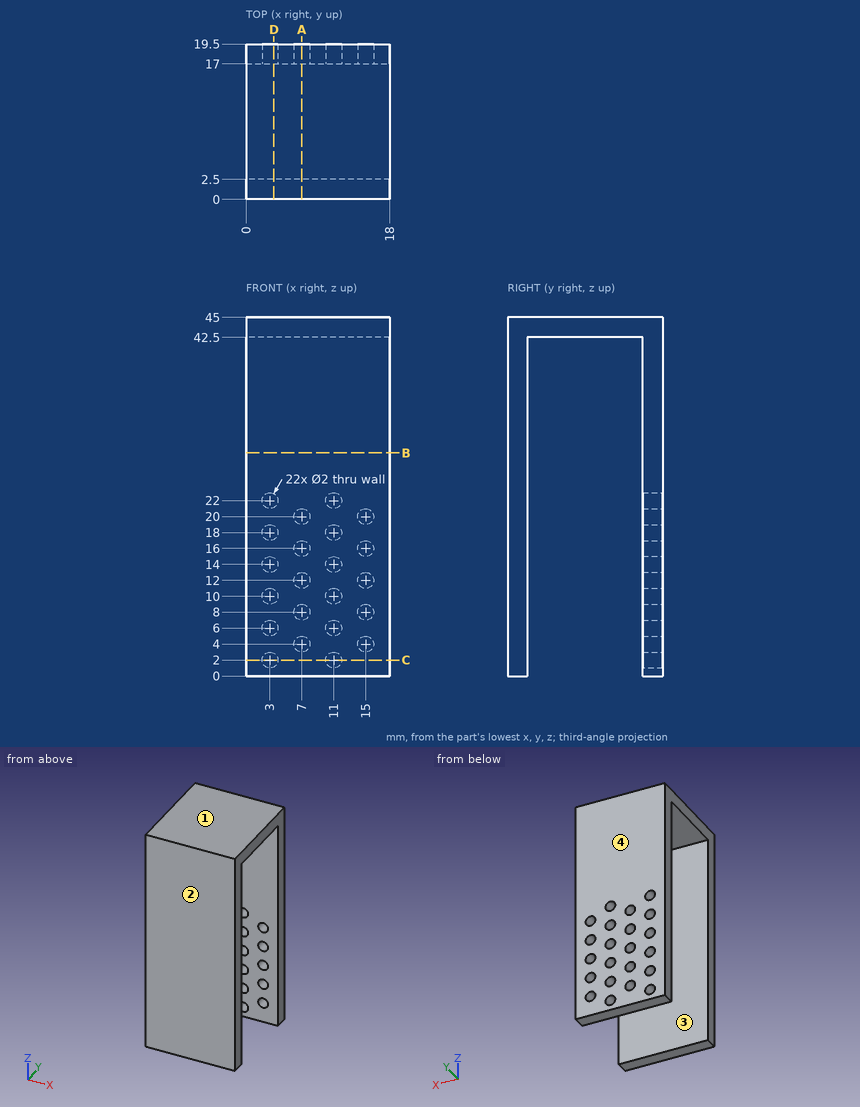
Print and shaded views of the part. All mm, measured from the part's lowest x, y and z. Coordinates: 2 decimals unless noted, no trailing zeros. Order: outer loops, then holes, each group sorted by start corner. A loop starts at its lowest first (then second) coordinate and runs counter-clockwise, first axis right, second up.
(1) Slice it at A-A, the plane x = 7. Write the cut outline in (y, z).
Check sheet entries:
outline: (0, 0) - (2.5, 0) - (2.5, 42.5) - (17, 42.5) - (17, 21) - (19.5, 21) - (19.5, 45) - (0, 45) - close; (17, 0) - (19.5, 0) - (19.5, 3) - (17, 3) - close; (17, 5) - (19.5, 5) - (19.5, 7) - (17, 7) - close; (17, 9) - (19.5, 9) - (19.5, 11) - (17, 11) - close; (17, 13) - (19.5, 13) - (19.5, 15) - (17, 15) - close; (17, 17) - (19.5, 17) - (19.5, 19) - (17, 19) - close
(2) Slice it at C-C, the plane z = 2. Write the cut outline in (x, y).
Check sheet entries:
outline: (0, 0) - (18, 0) - (18, 2.5) - (0, 2.5) - close; (0, 17) - (2, 17) - (2, 19.5) - (0, 19.5) - close; (4, 17) - (10, 17) - (10, 19.5) - (4, 19.5) - close; (12, 17) - (18, 17) - (18, 19.5) - (12, 19.5) - close
(3) Probe L1, parallel to X at y = 17.95, z = 6; L2, parallel to X at y = 17.9, z = 20; L3, parallel to Y at x = 7.5, z = 10. List the from-to ranges inside material, lowest first.
Check sheet entries:
L1: x = 0 to 2, 4 to 10, 12 to 18
L2: x = 0 to 6, 8 to 14, 16 to 18
L3: y = 0 to 2.5, 17 to 19.5
(4) Slice it at B-B, the plane z = 28. Write the cut outline in (x, y), and give its area (3 significant figures).
Check sheet entries:
outline: (0, 0) - (18, 0) - (18, 2.5) - (0, 2.5) - close; (0, 17) - (18, 17) - (18, 19.5) - (0, 19.5) - close
area: 90.0 mm2
(5) Pull direction Y, two halves, no side cores. Call the marked faces 1, 2, 3 and 4: pulls with the +Y half, pulls with the -Y half, needs draft (parallel to the pull), parting line crosses it, or undercut.
Check sheet entries:
face 1: needs draft
face 2: pulls with the -Y half
face 3: undercut
face 4: pulls with the +Y half
(6) Pin check, flat tips, straight feed: pin 1 Ø2 at (x, y) = (2, 14.5) entering from -Z; pin 2 Ø1.2 at (x, z) = (15, 16) entering from +Y. Stop position of each tip, or through.
Check sheet entries:
pin 1: stops at z = 42.5
pin 2: stops at y = 2.5
(7) Slice it at D-D, the plane x = 3.5. State how many separate pieces and enclosed holes the cut face has, and give its area (3 significant figures).
Check sheet entries:
separate pieces: 7
enclosed holes: 0
area: 235 mm2
